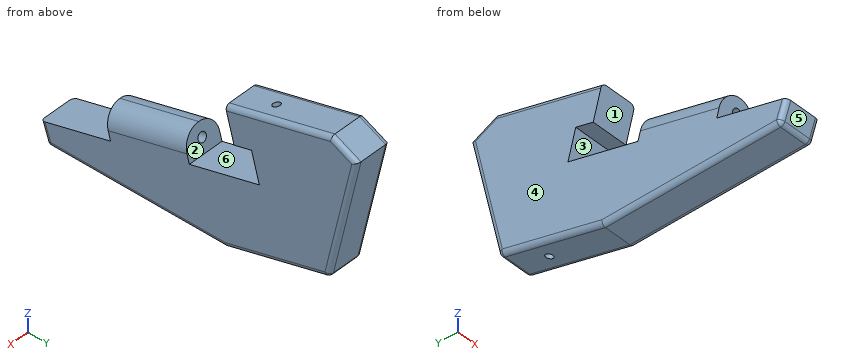
```python
from build123d import *

# Parameters (mm, degrees)
F1_DEPTH = 20
F3_D     = 10
F3_DEPTH = 90
F3_TIP   = 3.0043030951
F4_R     = 19.99999
F5_R     = 5
F7_D     = 8


# Not quite as in the source:
# - a fillet or chamfer is up to 0.001 mm smaller than in the source, because OpenCascade refuses the exact size


with BuildPart() as f1:
    # F0 (on Right) → F1 (new body, symmetric)
    with BuildSketch(Plane.YZ):
        Polygon((55.3865908633, 32.2499277236), (-31.5467335027, 8.9562136644), (-23.7821621496, -20.0215611243), (-101.0562282528, -40.7270847325), (-93.3750867844, -62.9337131977), (103.556553434, -62.9337131977), (217.0635979758, -32.5195922775), (248.1942623854, 104.8115119338), (219.449320977, 118.5184651202), (102.765125102, 87.253029066), (112.5305330656, 50.8080303895), (131.8490495913, 55.9844112915), (140.4252283195, 23.9776765432), (63.1511622164, 3.272152935), align=None)
    extrude(amount=F1_DEPTH, both=True)

    # F3
    with Locations(Plane(origin=(0, -27.1944496451, -7.286730821), x_dir=(1, 0, 0), z_dir=(0, -0.9659258263, -0.2588190451))):
        with Locations((0, 1.8159335255)):
            Hole(F3_D / 2, depth=F3_DEPTH)
            with Locations((0, 0, -(F3_DEPTH + F3_TIP / 2))):  # 118° drill point
                Cone(0, F3_D / 2, F3_TIP, mode=Mode.SUBTRACT)

    # F4 (radius 20 in the source; OpenCascade refuses exactly that, so slightly less here)
    f4_edges = [f1.edges().sort_by_distance(p)[0] for p in [
        (20, 11.919929, 20.603071),
        (-20, 11.919929, 20.603071),
    ]]
    fillet(f4_edges, radius=F4_R)

    # F5
    f5_edges = [f1.edges().sort_by_distance(p)[0] for p in [
        (-20, -97.215658, -51.830399),
        (20, -97.215658, -51.830399),
        (0, -93.375087, -62.933713),
        (20, 5.090733, -62.933713),
        (-20, 5.090733, -62.933713),
        (20, 160.310076, -47.726653),
        (-20, 160.310076, -47.726653),
        (0, 217.063598, -32.519592),
        (20, 232.62893, 36.14596),
        (-20, 232.62893, 36.14596),
        (-20, 233.821792, 111.664989),
        (20, 233.821792, 111.664989),
        (20, 161.107223, 102.885747),
        (-20, 161.107223, 102.885747),
    ]]
    fillet(f5_edges, radius=F5_R)

    # F7 (through all)
    with Locations(Plane(origin=(0, -14.9292991962, 55.7169031216), x_dir=(1, 0, 0), z_dir=(0, -0.2588190451, 0.9659258263))):
        with Locations((0, 161.846234043)):
            Hole(F7_D / 2)


solid = f1.part
```
CAD build for the part. Positions are in the model's coordinates, mm. Face numbers are marked on the shaded views. A direction names the side the tool comes from. Round coordinates to 2 decimals unless told otherwise and drop trailing zeros. Order: outer loops, then holes, each group sorted by start corner. A loop starts at its lowest first (then second) coordinate and runs counter-clockwise, first axis right, second up. Notation, with made-up numbers: (73, 66) - (121, 66) arc R20 cw to (121, 100) - close; hole circle Ø5 at (-26, 54). An arc over 180 degrees is marked (long way). Answer in a Markdown table with one row per item. Add a question column.
(1) Band-saw the part on C-C on y = 77. List the corners of the cut face in (x, z), and give its area (3 significant figures).
(2) Drop flat-ended pins along their axis: pin 1 Ø1.5 at (x, y) = (-12.5, 84) entering from +Z; pin 2 Ø1 at (x, z) = (-11.5, 37) entering from -Y; pin 3 Ø3 at (x, y) = (-15.5, 137) entering from -Z; pin 4 Ø1 at (y, z) = (63.5, 4.5) entering from +X. Give the stop position or say it passes through.
(3) Band-saw the part on B-B on x = 11.5. List the corners of the cut face in (y, z).
(4) 3-axis set-ups, long thin cutter, end or side, ignore diameter. For the marked faces 1, 2 and 3: which of +Z, -Z, +X, -X, +Y, -Y reach the whole face in a straight line?
(5) Mould opens along Y. For the marked faces 4, 5 and 6 say: +Y half, -Y half, draft (parallel to the pull), parting line (faces both ways), or undercut.
(6) Probe L1, parallel to Y at x = -3.5, z = 59; L2, parallel to Z at x = 3, y = 40; L3, parallel to Z at x = 10.5, y = 79. List the from-to ranges inside material, lowest first. Write a range as [from, to].
(7) Band-saw the part on A-A on y = -58. List the corners of the cut face in (x, z).
Data:
| question | item | result |
|---|---|---|
| 1 | outline | (-20, -57.93) arc R5 ccw to (-15, -62.93) - (15, -62.93) arc R5 ccw to (20, -57.93) - (20, 6.98) - (-20, 6.98) - close |
| 1 | area | 2,790 mm^2 |
| 2 | pin 1 | stops at z = 9.06 |
| 2 | pin 2 | stops at y = 136.8 |
| 2 | pin 3 | stops at z = -54.36 |
| 2 | pin 4 | passes through |
| 3 | outline | (-101.06, -40.73) - (-94.54, -59.57) arc R5 ccw to (-89.81, -62.93) - (103.56, -62.93) - (214.15, -33.3) arc R5 ccw to (217.73, -29.58) - (248.19, 104.81) - (219.45, 118.52) - (102.77, 87.25) - (112.53, 50.81) - (131.85, 55.98) - (140.43, 23.98) - (63.15, 3.27) - (56.33, 28.74) - (-30.61, 5.44) - (-23.78, -20.02) - close |
| 4 | face 1 | +X, -X, -Y |
| 4 | face 2 | +Z, +X, -X |
| 4 | face 3 | +X, -X |
| 5 | face 4 | draft |
| 5 | face 5 | -Y half |
| 5 | face 6 | undercut |
| 6 | L1 | y = [110.34, 149.74], [153.75, 237.81] |
| 6 | L2 | z = [-62.93, 8.46], [16.74, 27.89] |
| 6 | L3 | z = [-62.93, 7.52] |
| 7 | outline | (-20, -57.93) arc R5 ccw to (-15, -62.93) - (15, -62.93) arc R5 ccw to (20, -57.93) - (20, -29.19) - (-20, -29.19) - close |
